from build123d import *

# Parameters (mm, degrees)
SKETCH_R     = 4.3
PAD_DEPTH    = 9.2
POCKET_DEPTH = 4


with BuildPart() as part:
    # Sketch → Pad (new body)
    with BuildSketch(Plane.XY):
        Circle(SKETCH_R)
    extrude(amount=PAD_DEPTH)

    # Sketch003 → Pocket (cut)
    with BuildSketch(Plane.XY.offset(9.2)):
        Polygon((-3.5, 0), (-1.75, -3.031089), (1.75, -3.031089), (3.5, 0), (1.75, 3.031089), (-1.75, 3.031089), align=None)
    extrude(amount=-POCKET_DEPTH, mode=Mode.SUBTRACT)


solid = part.part
Check sheet for the modelled part. Datum: model origin and axes. Units: mm. A direction names the side the tool comes from. Give positions to 0.01 mm unless a question says otherwise; leave off trailing zeros. Order: outer loops, then holes, each group sorted by start corner. A loop starts at its lowest first (then second) coordinate and runs counter-clockwise, first axis right, second up. Notation, with made-up numbers: (80, -18.5) - (93, -18.5) arc R26 ccw to (93, 14.5) - close; hole circle Ø2 at (-16.5, 21). An arc over 180 degrees is marked (long way). Answer as CSV lines item,"result".
1. Section check A-A (z = 7.25). Record the boundary of the cut face in (x, y), then the cut area to 3 significant figures.
Result sheet:
outline,"circle Ø8.6 at (0, 0); hole (-3.5, 0) - (-1.75, -3.03) - (1.75, -3.03) - (3.5, 0) - (1.75, 3.03) - (-1.75, 3.03) - close"
area,"26.3 mm²"
2. Go/stop test with flat-tipped pins: P1, Ø1.5, axis at y = -2.5, z = 1.5, coming from the +X side; P2, Ø1, axis at y = 1, z = 3, coming from the +X side; P3, Ø1, axis at x = -3, z = 8, coming from the -Y side. Record where each tip stops, or that it passes through.
Result sheet:
P1,"x = 3.93"
P2,"x = 4.27"
P3,"y = -3.5"
3. Section check B-B (x = -3). Record the boundary of the cut face in (y, z), then the cut area to 3 significant figures.
Result sheet:
outline,"(-3.08, 0) - (3.08, 0) - (3.08, 9.2) - (0.87, 9.2) - (0.87, 5.2) - (-0.87, 5.2) - (-0.87, 9.2) - (-3.08, 9.2) - close"
area,"49.8 mm²"
4. Tool access check on faces 1 (the face through (0, -3.031, 7)), 2 (the face through (0, -3.2, 9.2)). Record the directions out of +Z, -Z, +X, -X, +Y, -Y that give a thin tool (end or side, any length) a straight path to the whole face; none if there is none.
Result sheet:
face 1,"+Z"
face 2,"+Z, +X, -X, +Y, -Y"
5. Scan lines: probe 1 along Y at (x, z) = (0, 8.5); probe 2 along Z at (x, y) = (-1, 0.75); probe 3 along X at (y, z) = (2, 6.5). Record each from-to range of solid material in increasing order. Write a range as from..to.
Result sheet:
probe 1,"-4.3..-3.03, 3.03..4.3"
probe 2,"0..5.2"
probe 3,"-3.81..-2.35, 2.35..3.81"
6. Section check C-C (y = 0.25). Record the boundary of the cut face in (x, z).
Result sheet:
outline,"(-4.29, 0) - (4.29, 0) - (4.29, 9.2) - (3.36, 9.2) - (3.36, 5.2) - (-3.36, 5.2) - (-3.36, 9.2) - (-4.29, 9.2) - close"
7. Mould release check, pull along Y, two halves, no side actions. Record for faces 3 (the face through (-2.61, 1.54, 7.23)), 4 (the face through (0, 0, 0)), 5 (the face through (-2.64, -1.49, 7.23)), 6 (the face through (-4.296, 0.189, 4.536)): released by +Y, released by -Y, zero draft, split by the parting line, or undercut.
Result sheet:
face 3,"undercut"
face 4,"zero draft"
face 5,"undercut"
face 6,"split by the parting line"
8. Section check D-D (z = 2.25). Record the boundary of the cut face in (x, y), then the cut area to 3 significant figures.
Result sheet:
outline,"circle Ø8.6 at (0, 0)"
area,"58.1 mm²"
